```python
from build123d import *

# Parameters (mm, degrees)
ESTRUSIONE_ESTRUSIONE1_DEPTH     = 5.05
FORO_FILETTATO_M3X0_5_1_D        = 2.5
FORO_FILETTATO_M2_5X0_45_1_D     = 2.05
FORO_FILETTATO_M2_5X0_45_1_DEPTH = 8
FORO_FILETTATO_M2_5X0_45_1_TIP   = 0.615882135
FORO_FILETTATO_M2_5X0_45_2_D     = 2.05
FORO_FILETTATO_M2_5X0_45_2_DEPTH = 9
FORO_FILETTATO_M2_5X0_45_2_TIP   = 0.615882135


with BuildPart() as part:
    # Schizzo1 → Estrusione-Estrusione1 (new body)
    with BuildSketch(Plane.XY):
        with BuildLine():
            Line((33.607852656, 57.990136231), (15.135967017, 57.990136231))
            ThreePointArc((15.135967017, 57.990136231), (14.569863255, 58.159527321), (14.189841424, 58.612020655))
            Line((14.189841424, 58.612020655), (13.644681905, 59.873833883))
            ThreePointArc((13.644681905, 59.873833883), (13.434009359, 60.124682426), (13.12017865, 60.218587695))
            Line((13.12017865, 60.218587695), (9.391909837, 60.218587695))
            Line((9.391909837, 60.218587695), (9.391909837, 24.597853141))
            ThreePointArc((9.391909837, 24.597853141), (9.577563808, 24.149644804), (10.025772145, 23.963990832))
            Line((10.025772145, 23.963990832), (18.675714063, 23.963990832))
            ThreePointArc((18.675714063, 23.963990832), (19.485298036, 23.822640523), (20.199085336, 23.415315332))
            Line((20.199085336, 23.415315332), (29.426699127, 15.777448227))
            ThreePointArc((29.426699127, 15.777448227), (30.330003033, 14.612437653), (30.65149016, 13.173739071))
            Line((30.65149016, 13.173739071), (30.65149016, 7.610644322))
            ThreePointArc((30.65149016, 7.610644322), (31.43997529, 5.707072826), (33.343546787, 4.918587695))
            Line((33.343546787, 4.918587695), (39.351909837, 4.918587695))
            Line((39.351909837, 4.918587695), (39.351909837, 60.218587695))
            Line((39.351909837, 60.218587695), (35.623641023, 60.218587695))
            ThreePointArc((35.623641023, 60.218587695), (35.309810314, 60.124682426), (35.099137768, 59.873833883))
            Line((35.099137768, 59.873833883), (34.553978249, 58.612020655))
            ThreePointArc((34.553978249, 58.612020655), (34.173956418, 58.159527321), (33.607852656, 57.990136231))
        make_face()
        with BuildLine():
            Line((31.031517622, 19.035447222), (21.858166203, 26.68561737))
            ThreePointArc((21.858166203, 26.68561737), (21.50418026, 27.348416385), (21.711670705, 28.070604932))
            Line((21.711670705, 28.070604932), (33.604209018, 43.239087362))
            ThreePointArc((33.604209018, 43.239087362), (34.717543506, 43.567327143), (35.391171024, 42.622085902))
            Line((35.391171024, 42.622085902), (35.391171024, 24.021384648))
            ThreePointArc((35.391171024, 24.021384648), (35.35046365, 23.738970664), (35.231655708, 23.479549344))
            Line((35.231655708, 23.479549344), (32.512468814, 19.26159802))
            ThreePointArc((32.512468814, 19.26159802), (31.822940625, 18.814892917), (31.031517622, 19.035447222))
        make_face(mode=Mode.SUBTRACT)
        with BuildLine():
            Line((15.844806521, 53.037240639), (31.196511098, 53.037240639))
            ThreePointArc((31.196511098, 53.037240639), (31.90361788, 52.74434742), (32.196511098, 52.037240639))
            Line((32.196511098, 52.037240639), (32.196511098, 48.227218639))
            ThreePointArc((32.196511098, 48.227218639), (32.142658979, 47.90348389), (31.986902723, 47.614616745))
            Line((31.986902723, 47.614616745), (18.775971342, 30.569600026))
            ThreePointArc((18.775971342, 30.569600026), (18.425692263, 30.284259301), (17.985579717, 30.182201919))
            Line((17.985579717, 30.182201919), (15.844806521, 30.182201919))
            ThreePointArc((15.844806521, 30.182201919), (15.13769974, 30.475095138), (14.844806521, 31.182201919))
            Line((14.844806521, 31.182201919), (14.844806521, 52.037240639))
            ThreePointArc((14.844806521, 52.037240639), (15.13769974, 52.74434742), (15.844806521, 53.037240639))
        make_face(mode=Mode.SUBTRACT)
    extrude(amount=ESTRUSIONE_ESTRUSIONE1_DEPTH)

    # Foro filettato M3x0.5-1 (through all)
    with Locations(Plane.XY.offset(5.05)):
        with Locations((35.391171024, 53.037240639), (12.391171024, 32.037240639), (35.391171024, 13.037240639)):
            Hole(FORO_FILETTATO_M3X0_5_1_D / 2)

    # Foro filettato M2.5x0.45-1
    with Locations(Plane(origin=(39.351909837, 0, 0), x_dir=(0, 0, -1), z_dir=(1, 0, 0))):
        with Locations((-2.525, 57.068587695), (-2.525, 8.068587695)):
            Hole(FORO_FILETTATO_M2_5X0_45_1_D / 2, depth=FORO_FILETTATO_M2_5X0_45_1_DEPTH)
            with Locations((0, 0, -(FORO_FILETTATO_M2_5X0_45_1_DEPTH + FORO_FILETTATO_M2_5X0_45_1_TIP / 2))):  # 118° drill point
                Cone(0, FORO_FILETTATO_M2_5X0_45_1_D / 2, FORO_FILETTATO_M2_5X0_45_1_TIP, mode=Mode.SUBTRACT)

    # Foro filettato M2.5x0.45-2
    with Locations(Plane.ZY.offset(-9.391909837)):
        with Locations((2.525, 57.068587695), (2.525, 27.068587695)):
            Hole(FORO_FILETTATO_M2_5X0_45_2_D / 2, depth=FORO_FILETTATO_M2_5X0_45_2_DEPTH)
            with Locations((0, 0, -(FORO_FILETTATO_M2_5X0_45_2_DEPTH + FORO_FILETTATO_M2_5X0_45_2_TIP / 2))):  # 118° drill point
                Cone(0, FORO_FILETTATO_M2_5X0_45_2_D / 2, FORO_FILETTATO_M2_5X0_45_2_TIP, mode=Mode.SUBTRACT)


solid = part.part
```
For this review, take the finished solid that the model builds, in its own axes (mm). A direction names the side the tool comes from. Give positions to 0.01 mm unless a question says otherwise; leave off trailing zeros. Order: outer loops, then holes, each group sorted by start corner. A loop starts at its lowest first (then second) coordinate and runs counter-clockwise, first axis right, second up.
1) For faces 1 (the face through (31.835, 18.817, 2.49)), 2 (the face through (38, 60.219, 2)), 3 (the face through (30.651, 10, 2)), list the 3-axis set-ups (+Z, -Z, +X, -X, +Y, -Y) from which the entire face can be reached by the end or side of a thin tool; tool diameter is ignored.
2) Take a section at C-C (y = 29). Give the boundary of the cut face in (x, z), then the cut area to 3 significant figures.
3) Insertion check: pin 1 (2 mm diameter, centred on x = 25.5, z = 2.5, fed in from +Y); pin 2 (2.5 mm diameter, centred on x = 23.5, z = 2.5, fed in from -Y); pin 3 (1.5 mm diameter, centred on x = 35.39, y = 13.04, fed in from -Z); pin 4 (1.2 mm diameter, centred on y = 8.07, z = 2.52, fed in from +X). Each pin has a flat end and moves straight along its axis. Give the tip position at first contact, or say it passes through.
4) Wall thickness on line 1 (X direction, y = 34.5, z = 4.35); line 2 (Y direction, x = 35, z = 0.95); line 3 (Y direction, x = 29.5, z = 2.9) (3 decimals): over which ranges is each line inside the solid? List them lowest first.
5) Take a section at A-A (x = 16.75). Give the boundary of the cut face in (y, z) (3 decimals), then the cut area to 3 significant figures.
6) Take a section at D-D (x = 22.75). Give the boundary of the cut face in (y, z).
7) Take a section at B-B (x = 12). Give the boundary of the cut face in (y, z) (3 decimals), then the cut area to 3 significant figures.
8) The part is to be moulded in two halves that separate along Z. For faces 4 (the face through (15.146, 30.467, 2.49)), 5 (the face through (27, 39, 5.05)), 6 (the face through (30.843, 8.245, 2.548)), 7 (the face through (27, 39, 0)), say which applies: released by +Z, released by -Z, zero draft, split by the parting line, or undercut.
Derived:
1. face 1: +Z, -Z
1. face 2: +Z, -Z, +X, -X, +Y
1. face 3: +Z, -Z, -X, -Y
2. outline: (9.39, 0) - (22.44, 0) - (22.44, 5.05) - (9.39, 5.05) - close; (35.39, 0) - (39.35, 0) - (39.35, 5.05) - (35.39, 5.05) - close
2. area: 85.9 mm2
3. pin 1: stops at y = 57.99
3. pin 2: stops at y = 19.65
3. pin 3: passes through
3. pin 4: stops at x = 31.1
4. line 1: x = 9.39 to 14.84, 21.82 to 26.75, 35.39 to 39.35
4. line 2: y = 4.92 to 11.85, 14.22 to 23.12, 43.42 to 51.85, 54.22 to 59.64
4. line 3: y = 15.715 to 20.313, 38.004 to 44.406, 53.037 to 57.99
5. outline: (23.964, 0) - (30.182, 0) - (30.182, 5.05) - (23.964, 5.05) - close; (53.037, 0) - (57.99, 0) - (57.99, 2.076) arc R1.025 cw (long way) to (57.99, 2.974) - (57.99, 5.05) - (53.037, 5.05) - close; hole circle Ø2.05 at (27.069, 2.525)
5. area: 49.9 mm2
6. outline: (21.3, 0) - (25.94, 0) - (25.94, 5.05) - (21.3, 5.05) - close; (29.39, 0) - (35.7, 0) - (35.7, 5.05) - (29.39, 5.05) - close; (53.04, 0) - (57.99, 0) - (57.99, 5.05) - (53.04, 5.05) - close
7. outline: (23.964, 0) - (30.85, 0) - (30.85, 5.05) - (23.964, 5.05) - close; (33.224, 0) - (60.219, 0) - (60.219, 5.05) - (33.224, 5.05) - close; hole circle Ø2.05 at (27.069, 2.525); hole circle Ø2.05 at (57.069, 2.525)
7. area: 164 mm2
8. face 4: zero draft
8. face 5: released by +Z
8. face 6: undercut
8. face 7: released by -Z
